from build123d import *

# Parameters (mm, degrees)
SKETCH_1_W      = 220
SKETCH_1_H      = 93
EXTRUDE_1_DEPTH = 5
FILLET_1_R      = 30
EXTRUDE_2_DEPTH = 5


with BuildPart() as part:
    # 草圖1 → 填料-伸長1 (new body)
    with BuildSketch(Plane(origin=(0, 0, 0), x_dir=(1, 0, 0), z_dir=(0, 1, 0))):
        Rectangle(SKETCH_1_W, SKETCH_1_H)
    extrude(amount=EXTRUDE_1_DEPTH)

    # 圓角1
    fillet_1_edges = [part.edges().sort_by_distance(p)[0] for p in [
        (110, 2.5, 46.5),
        (-110, 2.5, 46.5),
        (-110, 2.5, -46.5),
        (110, 2.5, -46.5),
    ]]
    fillet(fillet_1_edges, radius=FILLET_1_R)

    # 草圖2 → 填料-伸長2 (add)
    with BuildSketch(Plane.XZ):
        with BuildLine():
            Line((-80, -42), (80, -42))
            ThreePointArc((80, -42), (98.03122292, -34.53122292), (105.5, -16.5))
            Line((105.5, -16.5), (105.5, 16.5))
            ThreePointArc((105.5, 16.5), (98.03122292, 34.53122292), (80, 42))
            Line((80, 42), (-80, 42))
            ThreePointArc((-80, 42), (-98.03122292, 34.53122292), (-105.5, 16.5))
            Line((-105.5, 16.5), (-105.5, -16.5))
            ThreePointArc((-105.5, -16.5), (-98.03122292, -34.53122292), (-80, -42))
        make_face()
        with BuildLine():
            Line((-80, -36.5), (80, -36.5))
            ThreePointArc((80, -36.5), (94.142135624, -30.642135624), (100, -16.5))
            Line((100, -16.5), (100, 16.5))
            ThreePointArc((100, 16.5), (94.142135624, 30.642135624), (80, 36.5))
            Line((80, 36.5), (-80, 36.5))
            ThreePointArc((-80, 36.5), (-94.142135624, 30.642135624), (-100, 16.5))
            Line((-100, 16.5), (-100, -16.5))
            ThreePointArc((-100, -16.5), (-94.142135624, -30.642135624), (-80, -36.5))
        make_face(mode=Mode.SUBTRACT)
    extrude(amount=EXTRUDE_2_DEPTH)


solid = part.part
Design review of the part built by this model. Coordinates are the model's own, in mm. A direction names the side the tool comes from. Round coordinates to 2 decimals unless told otherwise and drop trailing zeros. Order: outer loops, then holes, each group sorted by start corner. A loop starts at its lowest first (then second) coordinate and runs counter-clockwise, first axis right, second up. Notation, with made-up numbers: M 29.25,30.5 L 71.25,30.5 A20 cw 71.25,55.5 Z; hole C 85,-7 d5. An arc over 180 degrees is marked long. Answer as CSV lines item,"result". Start each with the question number.
1) Tool access review of faces 1 (the face through (97.83, -2.46, -34.73)), 2 (the face through (-1, -2, -42)), 3 (the face through (-94.297, -2.465, -30.486)), 4 (the face through (-105.5, -2, 0)): name each direction out of +Z, -Z, +X, -X, +Y, -Y from which nothing blocks a thin tool from reaching the whole face with its end or side.
2) For pin 1 Ø5.5 at (y, z) = (-3.5, 6.5) entering from -X; pin 2 Ø1.5 at (x, y) = (15.5, -3.5) entering from -Z; pin 3 Ø4 at (y, z) = (-3, -6.5) entering from +X; pin 4 Ø5.5 at (x, y) = (-14, -2) entering from -Z, all flat-tipped, find the tip position at first contact; note any pin that passes through.
3) Add section C-C (x = 2.5). Give the boundary of the cut face in (y, z).
4) Wall thickness on line 1 along Z through (x, y) = (-12.5, -1); line 2 along Y through (x, z) = (15, 32); line 3 along X through (y, z) = (-2.5, -17): over which ranges is each line inside the solid? List them lowest first. Write a range as [from, to].
5) Add section A-A (y = -3.5). Give the boundary of the cut face in (x, z), then the cut area to 3 significant figures.
6) Add section B-B (z = -13.5). Give the boundary of the cut face in (x, y), then the cut area to 4 significant figures.
7) The part is to be moulded in two halves that separate along X. For faces 5 (the face through (-1, -2, -36.5)), 6 (the face through (-97.83, -2.46, 34.73)), 7 (the face through (110, 2, 0)), say which applies: +X half, -X half, draft (parallel to the pull), parting line (faces both ways), or undercut.
Resolved:
1,face 1,"-Z, +X, -Y"
1,face 2,"-Z, +X, -X, -Y"
1,face 3,"-Y"
1,face 4,"+Z, -Z, -X, -Y"
2,pin 1,"x = -105.5"
2,pin 2,"z = -42"
2,pin 3,"x = 105.5"
2,pin 4,"z = -46.5"
3,outline,"M -5,-42 L 0,-42 L 0,-46.5 L 5,-46.5 L 5,46.5 L 0,46.5 L 0,42 L -5,42 L -5,36.5 L 0,36.5 L 0,-36.5 L -5,-36.5 Z"
4,line 1,"[-42, -36.5], [36.5, 42]"
4,line 2,"[0, 5]"
4,line 3,"[-105.5, -99.99], [99.99, 105.5]"
5,outline,"M -105.5,-16.5 A25.5 ccw -80,-42 L 80,-42 A25.5 ccw 105.5,-16.5 L 105.5,16.5 A25.5 ccw 80,42 L -80,42 A25.5 ccw -105.5,16.5 Z; hole M -100,-16.5 A20 ccw -80,-36.5 L 80,-36.5 A20 ccw 100,-16.5 L 100,16.5 A20 ccw 80,36.5 L -80,36.5 A20 ccw -100,16.5 Z"
5,area,"2,910 mm^2"
6,outline,"M -110,0 L -105.5,0 L -105.5,-5 L -100,-5 L -100,0 L 100,0 L 100,-5 L 105.5,-5 L 105.5,0 L 110,0 L 110,5 L -110,5 Z"
6,area,"1,155 mm^2"
7,face 5,"undercut"
7,face 6,"-X half"
7,face 7,"+X half"
